Autodesk Inventor part; units mm, degrees
ref_plane "工作平面1" through (0, 0, 0) normal (0, 0, 1) x (1, 0, 0)
ref_plane "工作平面2" through (-32.5, 0, 6) normal (0, 0, 1) x (1, 0, 0)
ref_plane "工作平面3" through (-32.5, 0, 4) normal (0, 0, 1) x (1, 0, 0)
ref_plane "工作平面1" through (0, 0, 0) normal (0, 0, 1) x (1, 0, 0)
sketch "草图1" plane through (0, 0, 0) normal (0, 0, 1) x (1, 0, 0)
  arc A0 (-32.5, -65) -> (-32.5, 65) centre (-32.5, 0) ccw construction
  line L0 (-32.5, 40) -> (-32.5, 65) construction
  arc A1 (-32.5, -40) -> (-32.5, 40) centre (-32.5, 0) ccw construction
  line L1 (-32.5, -65) -> (-32.5, -40) construction
  circle A2 centre (-32.5, 0) radius 65
  circle A3 centre (-32.5, 0) radius 40
  circle A4 centre (-32.5, 0) radius 52.5 construction
  circle A5 centre (-85, 0) radius 5.5
  line L2 (-123.5, 0) -> (58.5, 0) construction
  circle A6 centre (-58.75, -45.4663) radius 5.5
  circle A7 centre (-6.25, -45.4663) radius 5.5
  circle A8 centre (20, 0) radius 5.5
  circle A9 centre (-6.25, 45.4663) radius 5.5
  circle A10 centre (-58.75, 45.4663) radius 5.5
  circle A11 centre (-32.5, 0) radius 35
  point P0 (0, 0)
  dimension "d0" = 105
  dimension "d1" = 11
  dimension "d4" = 360
  dimension "d6" = 70
extrude "拉伸1" add sketch "草图1" along normal blind 12 contours A2 | A3 | A11
sketch "草图2" plane through (-32.5, 0, 0) normal (0, 0, -1) x (-1, 0, 0)
  circle A0 centre (0, 0) radius 65 construction
  circle A1 centre (0, 0) radius 35
  circle A2 centre (0, 0) radius 40
  point P0 (-32.5, 0)
  dimension "d9" = 70
  dimension "d10" = 80
extrude "拉伸2" add sketch "草图2" along normal blind 20
sketch "草图3" plane through (-32.5, 0, 12) normal (0, 0, 1) x (1, 0, 0)
  circle A0 centre (0, 0) radius 18 construction
  circle A1 centre (0, 0) radius 19
  point P0 (32.5, 0)
  dimension "d23" = 38
extrude "拉伸3" cut sketch "草图3" against normal up to surface (12 mm away)
sketch "草图4" plane through (-32.5, 0, 12) normal (0, 0, 1) x (1, 0, 0)
  line L0 (-91, 0) -> (91, 0) construction
  circle A0 centre (0, 0) radius 65 construction
  line L1 (0, -101.0835) -> (0, 92.1895) construction
  circle A1 centre (0, 0) radius 40
  circle A2 centre (-52.5, 0) radius 5.5 construction
  circle A3 centre (0, 0) radius 19
  point P0 (32.5, 0)
  dimension "d16" = 80
extrude "拉伸4" cut sketch "草图4" against normal blind 1
fillet "圆角1" radius 1 1 edges at (-72.5, 0, 11)
ref_plane "工作平面2" through (-32.5, 0, 6) normal (0, 0, 1) x (1, 0, 0)
sketch "草图5" plane through (-32.5, 0, 0) normal (0, 0, -1) x (-1, 0, 0)
  circle A0 centre (0, 0) radius 40
  circle A1 centre (0, 0) radius 39
  point P0 (-32.5, 0)
  dimension "d20" = 1
extrude "拉伸5" cut sketch "草图5" along normal blind 2
sketch "草图6" plane through (-32.5, 0, 0) normal (0, 0, -1) x (-1, 0, 0)
  circle A0 centre (0, 0) radius 19
  circle A1 centre (0, 0) radius 35
  point P0 (-32.5, 0)
extrude "拉伸6" add sketch "草图6" along normal blind 3
ref_plane "工作平面3" through (-32.5, 0, 4) normal (0, 0, 1) x (1, 0, 0)
sketch "草图7" plane through (-32.5, 0, 4) normal (0, 0, 1) x (1, 0, 0)
  circle A0 centre (0, 0) radius 19 construction
  circle A1 centre (0, 0) radius 20.4
  point P0 (32.5, 0)
  dimension "d27" = 40.8
extrude "拉伸7" cut sketch "草图7" against normal mid plane 2.65
properties part number "轴承端盖1"
Read the model definition and answer for the solid it produces. Units are mm, in the model's axes. A direction names the side the tool comes from. Give positions to 0.01 mm unless a question says otherwise; leave off trailing zeros. Write each loop counter-clockwise with the first axis right and the second up, starting at its lowest first coordinate (ties: lowest second). Pieces come first, ordered by that corner, then holes. Notation, with made-up numbers: (-10.75, 81.5) - (-4.75, 81.5) arc R31 ccw to (-4.75, 112.5) - close; hole circle Ø8 at (31, 25.5). An arc over 180 degrees is marked (long way). Write item = value, one per line. Start each with the question number.
Item 1: Find section D-D (z = -4.5). Give the vertices of the cut face in (x, y).
Item 2: Find section B-B (y = 0). State how many separate pieces and enclosed holes the cut face has, then the cut area to 3 significant figures.
Item 3: A tool of negligible diameter and unlimited length cuts with its end or side. For faces 1 (the cylindrical face through (-36.619, -18.548, 8.202)), 2 (the cylindrical face through (-13.656, -7.813, 4.019)), 3 (the cylindrical face through (7.46, -1.76, -10.87)), from which of +Z, -Z, +X, -X, +Y, -Y can it reach the whole face along a straight path? Write none if from no direction.
Item 4: Find the intervals of material crossed by probe 1 along Y at (x, z) = (-6.5, 4); probe 2 along Y at (x, z) = (-6.25, 4.5); probe 3 along Z at (x, y) = (-55.5, 53), in increasing order. Write a range as [from, to].
Item 5: Each of these flat-tipped pins is pushed along its axis until it touches: P1, Ø23, axis at x = -32.5, y = 0, coming from the -Z side; P2, Ø8, axis at x = 10.5, z = 7, coming from the -Y side; P3, Ø8, axis at x = -51.5, z = -2, coming from the +Y side; P4, Ø6, axis at y = 38, z = 0.5, coming from the +X side. Where does it stop, or does it pass through?
Item 6: Find section C-C (z = 8.5). Give the vertices of the cut face in (x, y), then the cut area to 3 significant figures.
Item 7: The mould has two halves that part along Z. Classify faces 4 (the flat face through (-42, -17, 11)), 5 (the cylindrical face through (-6.97, -50.92, 5.92)), 6 (the flat face through (-42, 17, 5.325)), 7 (the flat face through (-48, -15, -3)): +Z half, -Z half, draft (parallel to the pull), parting line (faces both ways), or undercut.
Response:
q1.outline = circle Ø80 at (-32.5, 0); hole circle Ø70 at (-32.5, 0)
q2.separate_pieces = 4
q2.enclosed_holes = 0
q2.area = 1,080 mm²
q3.face_1 = +Z, -Z
q3.face_2 = none
q3.face_3 = -Z
q4.probe_1 = [-59.57, -50.96], [-39.97, 39.97], [50.96, 59.57]
q4.probe_2 = [-59.46, -50.97], [-39.97, 39.97], [50.97, 59.46]
q4.probe_3 = [0, 12]
q5.P1 = through
q5.P2 = -52
q5.P3 = 63.12
q5.P4 = 22.27
q6.outline = circle Ø130 at (-32.5, 0); hole circle Ø11 at (-85, 0); hole circle Ø11 at (-58.75, -45.47); hole circle Ø11 at (-58.75, 45.47); hole circle Ø38 at (-32.5, 0); hole circle Ø11 at (-6.25, -45.47); hole circle Ø11 at (-6.25, 45.47); hole circle Ø11 at (20, 0)
q6.area = 11,600 mm²
q7.face_4 = +Z half
q7.face_5 = draft
q7.face_6 = undercut
q7.face_7 = -Z half
